Could you check a few things on this drawing? It's one solid part, dimensions in mm from its lowest x, y, z. Give positions to 0.01 mm unless a question says otherwise; leave off trailing zeros. Write each loop counter-clockwise with the first axis right and the second up, starting at its lowest first coordinate (ties: lowest second). Pieces come first, ordered by that corner, then holes. Notation, with made-up numbers: (83.25, -17.5) - (133.25, -17.5) arc R9 cw to (133.25, -8.5) - close; hole circle Ø11 at (69, 89.25). An arc over 180 degrees is marked (long way). One line per item, written item: value. Start each with the question number.
1) Imagine slicing it at A-A on y = 2. Write out the boundary of the cut face in (x, z).
2) Imagine slicing it at C-C on x = 34. Write out the boundary of the cut face in (y, z).
3) Imagine slicing it at B-B on z = 42.5. Write out the boundary of the cut face in (x, y), plus the area to 3 significant figures.
4) I'm going to push flat-ended pins straight in: P1, Ø8.5, axis at x = 422.148, z = 12.7, coming from the -Y side; P2, Ø4, axis at y = 8.5, z = 42, coming from the -X side. Where does each tip first touch, or does it pass through?
5) Please list where these lines run through material, in increasing order: L1, parallel to X at y = 10, z = 495.3 (3 decimals); L2, parallel to Z at x = 424, y = 3.75; L3, parallel to X at y = 3.75, z = 35. Write a range as [from, to].
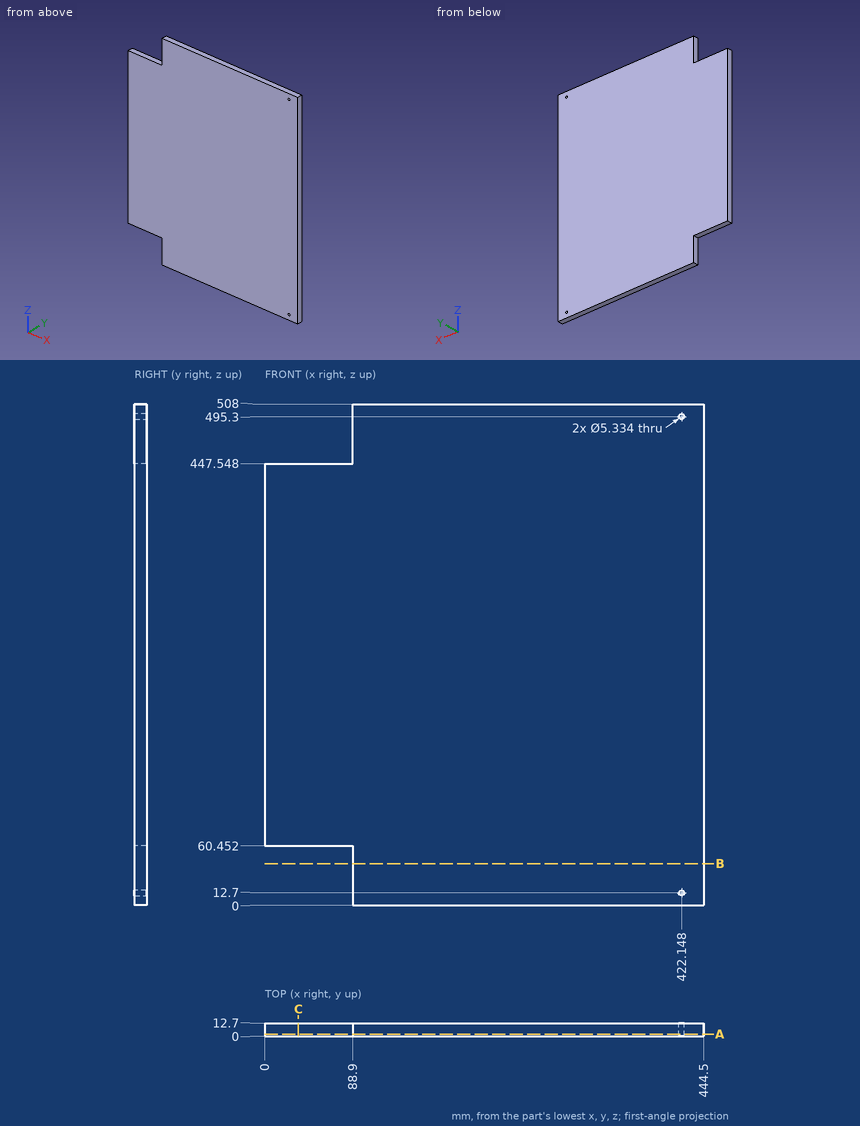
Numbers:
1. outline: (0, 60.45) - (88.9, 60.45) - (88.9, 0) - (444.5, 0) - (444.5, 508) - (88.9, 508) - (88.9, 447.55) - (0, 447.55) - close; hole circle Ø5.33 at (422.15, 12.7); hole circle Ø5.33 at (422.15, 495.3)
2. outline: (0, 60.45) - (12.7, 60.45) - (12.7, 447.55) - (0, 447.55) - close
3. outline: (88.9, 0) - (444.5, 0) - (444.5, 12.7) - (88.9, 12.7) - close
3. area: 4,520 mm^2
4. P1: y = 0
4. P2: x = 88.9
5. L1: [88.9, 419.481], [424.815, 444.5]
5. L2: [0, 10.78], [14.62, 493.38], [497.22, 508]
5. L3: [88.9, 444.5]
